The listing builds one solid part. Answer for the finished solid, in the listing's coordinates (mm). Give positions to 0.01 mm unless a question says otherwise; leave off trailing zeros. Loops run counter-clockwise (first coordinate to the right, second up) from the corner with the lowest first, then second, coordinate; pieces in that order, holes last. Notation, with made-up numbers: (58.5, -28) - (92.5, -28) arc R28 ccw to (92.5, -6) - close; hole circle Ø5 at (73, 70.25). An arc over 180 degrees is marked (long way). Answer as CSV lines item,"result". Start each with the question number.
1) A cutting plane is placed at B-B (x = -5.75). Determine the outline of the cut face in (y, z).
2) A cutting plane is placed at C-C (z = 0.8). Determine the outline of the cut face in (x, y).
3) A flat-ended cylindrical pin translates along its axis: pin 1 (2.5 mm diameter, centred on x = 10, y = -10, fed in from +Z). Find the tip coordinate at first contact, or state that the pin passes through.
4) A cutting plane is placed at D-D (y = -9). Determine the outline of the cut face in (x, z), and give its area (3 significant figures).
5) For a pull along X with two mould halves and no side action, classify faces 1 (the face through (0, -13.5, 1)), 2 (the face through (-13.5, 0, 1)), 3 (the face through (4.57, 7.167, 0.74)) as pulls with the +X half, pulls with the -X half, needs draft (parallel to the pull), parting line crosses it, or undercut.
6) Find the intervals of material crossed by line 1 along Y through (x, z) = (-10.5, 0.5); line 2 along Y through (x, z) = (10, 0.5); line 3 along Y through (x, z) = (5.5, 1.4), in increasing order.
7) A cutting plane is placed at A-A (y = 0). Determine the outline of the cut face in (x, z), and give its area (3 significant figures).
```python
from build123d import *

# Parameters (mm, degrees)
F0_R     = 1.5
F0_R_2   = 8.5
F1_DEPTH = 1.5


with BuildPart() as f1:
    # F0 (on Top) → F1 (new body)
    with BuildSketch(Plane.XY):
        with BuildLine():
            ThreePointArc((13.5, 9.5), (12.328427, 12.328427), (9.5, 13.5))
            Line((9.5, 13.5), (-9.5, 13.5))
            ThreePointArc((-9.5, 13.5), (-12.328427, 12.328427), (-13.5, 9.5))
            Line((-13.5, 9.5), (-13.5, -9.5))
            ThreePointArc((-13.5, -9.5), (-12.328427, -12.328427), (-9.5, -13.5))
            Line((-9.5, -13.5), (9.5, -13.5))
            ThreePointArc((9.5, -13.5), (12.328427, -12.328427), (13.5, -9.5))
            Line((13.5, -9.5), (13.5, 9.5))
        make_face()
        with Locations((-10, -10)):
            Circle(F0_R, mode=Mode.SUBTRACT)
        with Locations((10, -10)):
            Circle(F0_R, mode=Mode.SUBTRACT)
        with Locations((-10, 10)):
            Circle(F0_R, mode=Mode.SUBTRACT)
        Circle(F0_R_2, mode=Mode.SUBTRACT)
        with Locations((10, 10)):
            Circle(F0_R, mode=Mode.SUBTRACT)
    extrude(amount=F1_DEPTH)


solid = f1.part
```
Ans:
1,outline,"(-13.5, 0) - (-6.26, 0) - (-6.26, 1.5) - (-13.5, 1.5) - close; (6.26, 0) - (13.5, 0) - (13.5, 1.5) - (6.26, 1.5) - close"
2,outline,"(-13.5, -9.5) arc R4 ccw to (-9.5, -13.5) - (9.5, -13.5) arc R4 ccw to (13.5, -9.5) - (13.5, 9.5) arc R4 ccw to (9.5, 13.5) - (-9.5, 13.5) arc R4 ccw to (-13.5, 9.5) - close; hole circle Ø3 at (-10, -10); hole circle Ø3 at (-10, 10); hole circle Ø17 at (0, 0); hole circle Ø3 at (10, -10); hole circle Ø3 at (10, 10)"
3,pin 1,"through"
4,outline,"(-13.5, 0) - (-11.12, 0) - (-11.12, 1.5) - (-13.5, 1.5) - close; (-8.88, 0) - (8.88, 0) - (8.88, 1.5) - (-8.88, 1.5) - close; (11.12, 0) - (13.5, 0) - (13.5, 1.5) - (11.12, 1.5) - close"
4,area,"33.8 mm2"
5,face 1,"needs draft"
5,face 2,"pulls with the -X half"
5,face 3,"undercut"
6,line 1,"-13.37 to -11.41, -8.59 to 8.59, 11.41 to 13.37"
6,line 2,"-13.47 to -11.5, -8.5 to 8.5, 11.5 to 13.47"
6,line 3,"-13.5 to -6.48, 6.48 to 13.5"
7,outline,"(-13.5, 0) - (-8.5, 0) - (-8.5, 1.5) - (-13.5, 1.5) - close; (8.5, 0) - (13.5, 0) - (13.5, 1.5) - (8.5, 1.5) - close"
7,area,"15.0 mm2"
